The listing builds one solid part. Answer for the finished solid, in the listing's coordinates (mm). Face numbers are marked on the shaded views. A direction names the side the tool comes from. Give positions to 0.01 mm unless a question says otherwise; leave off trailing zeros. Loops run counter-clockwise (first coordinate to the right, second up) from the corner with the lowest first, then second, coordinate; pieces in that order, holes last. Notation, with made-up numbers: (-19.5, 69) - (-1.5, 69) arc R20 cw to (-1.5, 102) - close; hole circle Ø6 at (30.25, 23). An arc over 180 degrees is marked (long way). Write item = value, one per line. Start each with the question number.
1) The part is cut by section A-A on x = 0. State how many separate pieces and enclosed holes the cut face has, plus the area to 3 significant figures.
2) The part is cut by section C-C on y = -22. Write down the section's boundary in (x, z) (1 decimal), plus the area to 3 significant figures.
3) Which of the six approach directions +Z, -Z, +X, -X, +Y, -Y give full straight-line access (tool end or side, diameter ignored) to the marked faces 1, 2, 3 and 4?
4) The part is cut by section D-D on z = -3. Write down the section's boundary in (x, y), plus the area to 3 significant figures.
5) Consider probe 1 along Z at (x, y) = (0, 4.65); probe 2 along X at (y, z) = (4.35, -19.05); probe 3 along Y at (x, z) = (-11, -19). Determine where each line is inside the solid, lowest interval first.
6) Flat-ended cylindrical pins translate along their axes: P1, Ø1.5, axis at x = 7.5, z = -12.5, coming from the -Y side; P2, Ø5, axis at y = -28.5, z = -11.5, coming from the -X side; P3, Ø5.5, axis at x = 0, z = -19.05, coming from the -Y side. Find the tip coordinate at first contact, or state that the pin passes through.
7) The mould has two halves that part along X. Classify the marked faces 5, 6 and 7: +X half, -X half, draft (parallel to the pull), parting line (faces both ways), or undercut.
8) The part is cut by section B-B on z = 19.05. Write down the section's boundary in (x, y) (3 decimals).
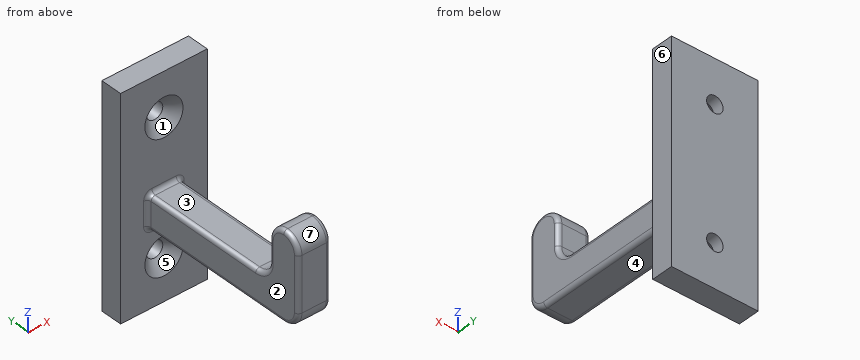
Autodesk Fusion 360 part; units mm, degrees
sketch "Sketch1" plane through (0, 0, 0) normal (0, 1, 0) x (1, 0, 0) in component "Component"
  line L0 (12.7, 31.75) -> (-12.7, 31.75)
  line L1 (-12.7, 31.75) -> (-12.7, -31.75)
  line L2 (-12.7, -31.75) -> (12.7, -31.75)
  line L3 (12.7, -31.75) -> (12.7, 31.75)
  line L4 (12.7, 31.75) -> (-12.7, -31.75) construction
  line L5 (-12.7, 31.75) -> (12.7, -31.75) construction
  dimension "d1" = 63.5
  dimension "d2" = 25.4
extrude "Extrude1" add sketch "Sketch1" along normal blind 6.35 in component "Component"
hole "Hole1" at (0, 0, 19.05) direction (0, 1, 0) diameter 4.826 end through all in component "Component"
mirror "Mirror1" about plane through (0, 0, 0) normal (0, 0, 1) of "Hole1" in component "Component"
sketch "Sketch2" plane through (0, 0, 0) normal (1, 0, 0) x (0, 1, 0) in component "Component"
  line L0 (0, -9.525) -> (-50.8, -9.525)
  line L1 (-50.8, -9.525) -> (-50.8, 15.875)
  line L2 (-50.8, 15.875) -> (-41.275, 15.875)
  line L3 (-41.275, 15.875) -> (-41.275, 0)
  line L4 (-41.275, 0) -> (0, 0)
  line L5 (0, 0) -> (0, -9.525)
  line L6 (0, 0) -> (-81.1043, 0) construction
  dimension "d11" = 9.525
  dimension "d12" = 9.525
  dimension "d13" = 50.8
  dimension "d14" = 25.4
extrude "Extrude2" add sketch "Sketch2" along normal mid plane 9.525 in component "Component"
fillet "Fillet1" radius 4.7625 4 edges at (0, -50.8, -9.525) (0, -41.275, 0) (0, -50.8, 15.875) (0, -41.275, 15.875) in component "Component"
fillet "Fillet2" radius 1.1906 14 edges at (4.7625, -18.2563, 0) (4.7625, -39.8801, 1.3949) (4.7625, -41.275, 7.9375) (4.7625, -46.0375, 15.875) (4.7625, -50.8, 3.175) (4.7625, -49.4051, -8.1301) (4.7625, -23.0187, -9.525) (-4.7625, -23.0187, -9.525) (-4.7625, -49.4051, -8.1301) (-4.7625, -50.8, 3.175) (-4.7625, -46.0375, 15.875) (-4.7625, -41.275, 7.9375) (-4.7625, -39.8801, 1.3949) (-4.7625, -18.2563, 0) in component "Component"
fillet "Fillet2" radius 1.1906 2 edges at (-4.7625, 0, -4.7625) (4.7625, 0, -4.7625) in component "Component"
chamfer "Chamfer1" distance 3.175 angle 45 2 edges at (0.8726, 0, 21.2997) (-0.8726, 0, -21.2997) in component "Component"
component "Component" placed x (1, 0, 0) y (0, 1, 0) z (0, 0, 1) at (0, 0, 0)
equation "d11 = ( 3 / 8 ) * 1 in"
equation "d15 = ( 3 / 8 ) * 1 in"
equation "d17 = ( 3 / 16 ) * 1 in"
equation "d18 = ( 3 / 64 ) * 1 in"
equation "d19 = ( 3 / 64 ) * 1 in"
Answer below:
q1.separate_pieces = 3
q1.enclosed_holes = 0
q1.area = 948 mm2
q2.outline = (-4.8, -8.3) arc R1.2 ccw to (-3.6, -9.5) - (3.6, -9.5) arc R1.2 ccw to (4.8, -8.3) - (4.8, -1.2) arc R1.2 ccw to (3.6, 0) - (-3.6, 0) arc R1.2 ccw to (-4.8, -1.2) - close
q2.area = 89.5 mm2
q3.face_1 = none
q3.face_2 = +Z, -Z, -X, -Y
q3.face_3 = +Z, +X, -X
q3.face_4 = -Z, +X, -X, -Y
q4.outline = (-12.7, 0) - (-5.95, 0) arc R1.19 cw to (-4.76, -1.19) - (-4.76, -49.61) arc R1.19 ccw to (-3.57, -50.8) - (3.57, -50.8) arc R1.19 ccw to (4.76, -49.61) - (4.76, -1.19) arc R1.19 cw to (5.95, 0) - (12.7, 0) - (12.7, 6.35) - (-12.7, 6.35) - close
q4.area = 645 mm2
q5.probe_1 = -31.75 to -21.46, -16.64 to 16.64, 21.46 to 31.75
q5.probe_2 = -12.7 to -2.41, 2.41 to 12.7
q5.probe_3 = 0 to 6.35
q6.P1 = 0
q6.P2 = -4.56
q6.P3 = 2.84
q7.face_5 = undercut
q7.face_6 = +X half
q7.face_7 = draft
q8.outline = (-12.7, 0) - (-5.588, 0) - (-2.413, 3.175) - (-2.413, 6.35) - (-12.7, 6.35) - close; (2.413, 3.175) - (5.588, 0) - (12.7, 0) - (12.7, 6.35) - (2.413, 6.35) - close
